Can you work these out from the model? Positions are in its coordinate system, mm. A direction names the side the tool comes from. Coordinates: 2 decimals unless noted, no trailing zeros. Write each loop counter-clockwise with the first axis right and the second up, starting at its lowest first coordinate (ties: lowest second). Pieces come first, ordered by that corner, then holes. Notation, with made-up numbers: M 70,81.25 L 99,81.25 A21 ccw 99,95.25 Z; hole C 88.5,84.5 d2. An arc over 180 degrees is marked long. Answer as a JSON object with one key per item and string values. Group by question number.
from build123d import *

# Parameters (mm, degrees)
PAD_DEPTH     = 7.5
SKETCH002_W   = 34
SKETCH002_H   = 6.8
PAD001_DEPTH  = 0.6
SKETCH001_W   = 35.08
SKETCH001_H   = 7.18
PAD002_DEPTH  = 14
PAD003_DEPTH  = 0.5
PAD004_DEPTH  = 0.5
SKETCH005_W   = 35.08
SKETCH005_H   = 7.18
SKETCH005_W_2 = 15.99
SKETCH005_H_2 = 4.6
PAD005_DEPTH  = 1
POCKET_DEPTH  = 16.5


with BuildPart() as part:
    # Sketch → Pad (new body)
    with BuildSketch(Plane.XY):
        Polygon((-20.01, 4), (-3.25, 4), (-3.25, 5), (3.25, 5), (3.25, 4), (20.01, 4), (20.01, -4), (-20.01, -4), align=None)
        Polygon((-19.01, 3), (-2.25, 3), (-2.25, 4), (2.25, 4), (2.25, 3), (19.01, 3), (19.01, -3), (-19.01, -3), align=None, mode=Mode.SUBTRACT)
    extrude(amount=-PAD_DEPTH)

    # Sketch002 → Pad001 (join)
    with BuildSketch(Plane.XY):
        Polygon((-20.01, 4), (-20.01, -4), (20.01, -4), (20.01, 4), (3.25, 4), (3.25, 5), (-3.25, 5), (-3.25, 4), align=None)
        Rectangle(SKETCH002_W, SKETCH002_H, mode=Mode.SUBTRACT)
    extrude(amount=PAD001_DEPTH)

    # Sketch001 → Pad002 (join)
    with BuildSketch(Plane.XY):
        Rectangle(SKETCH001_W, SKETCH001_H)
        with BuildLine():
            Line((16.54, 2.59), (16.54, -2.59))
            Line((16.54, -2.59), (8.82, -2.59))
            Line((8.82, -0.5), (8.82, -2.59))
            ThreePointArc((8.82, -0.5), (8.673553, -0.146447), (8.32, 0))
            Line((6.92, 0), (8.32, 0))
            ThreePointArc((6.92, 0), (6.566447, -0.146447), (6.42, -0.5))
            Line((6.42, -2.59), (6.42, -0.5))
            Line((6.42, -2.59), (-14.14, -2.59))
            Line((-14.14, -2.59), (-14.14, -0.5))
            ThreePointArc((-14.14, -0.5), (-14.286447, -0.146447), (-14.64, 0))
            Line((-14.64, 0), (-16.54, 0))
            Line((-16.54, 0), (-16.54, 2.59))
            Line((-16.54, 2.59), (8.96, 2.59))
            Line((8.96, 0.5), (8.96, 2.59))
            ThreePointArc((8.96, 0.5), (9.106447, 0.146447), (9.46, 0))
            Line((10.86, 0), (9.46, 0))
            ThreePointArc((10.86, 0), (11.213553, 0.146447), (11.36, 0.5))
            Line((11.36, 2.59), (11.36, 0.5))
            Line((11.36, 2.59), (16.54, 2.59))
        make_face(mode=Mode.SUBTRACT)
    extrude(amount=PAD002_DEPTH)

    # Sketch003 (on Face1 of Pad) → Pad003 (join)
    with BuildSketch(Plane(origin=(0, 4, 0), x_dir=(-1, 0, 0), z_dir=(0, 1, 0))):
        Polygon((15, -6), (16.5, -1.5), (13.5, -1.5), align=None)
    extrude(amount=PAD003_DEPTH)

    # Sketch004 (on Face33 of Pad003) → Pad004 (join)
    with BuildSketch(Plane.XZ.offset(3.59)):
        Polygon((16.568533, 6.35), (15.24, 12.7), (14.028533, 6.35), align=None)
    extrude(amount=PAD004_DEPTH)

    # Sketch005 → Pad005 (join)
    with BuildSketch(Plane.XY.offset(14)):
        Rectangle(SKETCH005_W, SKETCH005_H)
        with Locations((-8.445, 0)):
            Rectangle(SKETCH005_W_2, SKETCH005_H_2, mode=Mode.SUBTRACT)
        with Locations((8.445, 0)):
            Rectangle(SKETCH005_W_2, SKETCH005_H_2, mode=Mode.SUBTRACT)
    extrude(amount=PAD005_DEPTH)

    # Sketch006 → Pocket (cut, symmetric)
    with BuildSketch(Plane.YZ):
        Polygon((-3, 0), (-3, -1), (3, -1), (3, 0), (0, 3), align=None)
    extrude(amount=POCKET_DEPTH, both=True, mode=Mode.SUBTRACT)


solid = part.part
Q1. Please list where these lines run through material, in increasing order: L1, parallel to X at y = -1.5, z = 12.5; L2, parallel to Y at x = 17.5, z = -1.5; L3, parallel to Y at x = -15.5, z = 11.75.
Q2. Will these pins go through, and if not, where does the flat tip stop? pin 1 (1 mm diameter, centred on y = -2, z = 8, fed in from +X); pin 2 (1.7 mm diameter, centred on y = -1.5, z = 10.5, fed in from -X); pin 3 (8 mm diameter, centred on x = -0.5, z = 6.5, fed in from -Y).
Q3. On a 3-axis mill with a long thin cutter (end or side, diameter ignored), from which of +Z, -Z, +X, -X, +Y, -Y can I reach the whole of each face in a straight line? I mean faces 1 (the flat face through (-16.44, 0, 14.5)), 2 (the flat face through (-14.24, 4.25, -3.72)), 3 (the flat face through (-0.45, 0, 14.5)), 4 (the flat face through (-14.14, -2, 7)), 5 (the flat face through (0, 3.59, 8)). Say none if no direction works.
Q4. If we section it at B-B on x = -9.5: List the corners of the cut face in (y, z) for me, and give its area (3 significant figures).
Q5. If we section it at A-A on y = 1.5: List the corners of the cut face in (x, z) for me.
Q6. If we section it at D-D on x = -1.5: List the corners of the cut face in (y, z) for me, and give its area (3 significant figures).
Reply:
{
 "1": {"L1": "-17.54 to -14.14, 6.42 to 8.82, 16.54 to 17.54", "L2": "-4 to -3, 3 to 4", "L3": "-3.59 to 0, 2.59 to 3.59"},
 "2": {"pin 1": "x = 17.54", "pin 2": "x = -17.54", "pin 3": "y = -3.59"},
 "3": {"face 1": "+Z", "face 2": "-Z, +Y", "face 3": "+Z, -Z", "face 4": "-Z", "face 5": "+Z, +X, -X, +Y"},
 "4": {"outline": "M -4,-7.5 L -3,-7.5 L -3,0 L -2.59,0.41 L -2.59,14 L -2.3,14 L -2.3,15 L -3.59,15 L -3.59,0.6 L -4,0.6 Z; M 2.3,14 L 2.59,14 L 2.59,0.41 L 3,0 L 3,-7.5 L 4,-7.5 L 4,0.6 L 3.59,0.6 L 3.59,15 L 2.3,15 Z", "area": "45.9 mm^2"},
 "5": {"outline": "M -20.01,-7.5 L -19.01,-7.5 L -19.01,0 L -16.54,0 L -16.54,14 L -16.44,14 L -16.44,15 L -17.54,15 L -17.54,0.6 L -20.01,0.6 Z; M -0.45,14 L 0.45,14 L 0.45,15 L -0.45,15 Z; M 8.96,1.5 L 11.36,1.5 L 11.36,14 L 8.96,14 Z; M 16.44,14 L 16.54,14 L 16.54,0 L 19.01,0 L 19.01,-7.5 L 20.01,-7.5 L 20.01,0.6 L 17.54,0.6 L 17.54,15 L 16.44,15 Z"},
 "6": {"outline": "M -4,-7.5 L -3,-7.5 L -3,0 L -2.59,0.41 L -2.59,14 L -2.3,14 L -2.3,15 L -3.59,15 L -3.59,0.6 L -4,0.6 Z; M 2.3,14 L 2.59,14 L 2.59,0.41 L 3,0 L 4,0 L 4,-7.5 L 5,-7.5 L 5,0.6 L 3.59,0.6 L 3.59,15 L 2.3,15 Z", "area": "46.5 mm^2"}
}
